```python
from build123d import *

# Parameters (mm, degrees)
CROQUIS1_W              = 200
CROQUIS1_H              = 200
CROQUIS1_R              = 2.5
SALIENTE_EXTRUIR1_DEPTH = 0.5
CORTAR_EXTRUIR1_DEPTH   = 10


with BuildPart() as part:
    # Croquis1 → Saliente-Extruir1 (new body)
    with BuildSketch(Plane(origin=(0, 0, 0), x_dir=(1, 0, 0), z_dir=(0, 1, 0))):
        with Locations((100, 100)):
            Rectangle(CROQUIS1_W, CROQUIS1_H)
        with Locations(Location((15, 185, 0), (0, 0, 270))):
            Circle(CROQUIS1_R, mode=Mode.SUBTRACT)
        with Locations(Location((185, 185, 0), (0, 0, 270))):
            Circle(CROQUIS1_R, mode=Mode.SUBTRACT)
        with Locations(Location((185, 15, 0), (0, 0, 270))):
            Circle(CROQUIS1_R, mode=Mode.SUBTRACT)
        with Locations(Location((15, 15, 0), (0, 0, 270))):
            Circle(CROQUIS1_R, mode=Mode.SUBTRACT)
    extrude(amount=SALIENTE_EXTRUIR1_DEPTH)

    # Croquis2 → Cortar-Extruir1 (cut)
    with BuildSketch(Plane(origin=(0, 0.5, 0), x_dir=(1, 0, 0), z_dir=(0, 1, 0))):
        Polygon((50, 148), (50, 100), (50, 52), (52, 52), (52, 50), (100, 50), (148, 50), (148, 52), (150, 52), (150, 100), (150, 148), (148, 148), (148, 150), (100, 150), (52, 150), (52, 148), align=None)
    extrude(amount=-CORTAR_EXTRUIR1_DEPTH, mode=Mode.SUBTRACT)


solid = part.part
```
Geometry check sheet. Reference: the model listing, model coordinates, mm. Give positions to 0.01 mm unless a question says otherwise; leave off trailing zeros. Write each loop counter-clockwise with the first axis right and the second up, starting at its lowest first coordinate (ties: lowest second). Pieces come first, ordered by that corner, then holes. Notation, with made-up numbers: (-37, 7) -> (-30, 7) arc R24 ccw to (-30, 41) -> close; hole circle Ø10 at (-34, -9.5). An arc over 180 degrees is marked (long way). One line per question, with ' | ' between items.
Item 1: Sectioned sample at A-A, the plane z = -106. Record the boundary of the cut face in (x, y).
Determined:
outline: (0, 0) -> (50, 0) -> (50, 0.5) -> (0, 0.5) -> close; (150, 0) -> (200, 0) -> (200, 0.5) -> (150, 0.5) -> close
Item 2: Sectioned sample at C-C, the plane y = 0.3. Record the boundary of the cut face in (x, z), plus the area to 3 significant figures.
Determined:
outline: (0, -200) -> (200, -200) -> (200, 0) -> (0, 0) -> close; hole circle Ø5 at (15, -185); hole circle Ø5 at (15, -15); hole (50, -148) -> (52, -148) -> (52, -150) -> (148, -150) -> (148, -148) -> (150, -148) -> (150, -52) -> (148, -52) -> (148, -50) -> (52, -50) -> (52, -52) -> (50, -52) -> close; hole circle Ø5 at (185, -185); hole circle Ø5 at (185, -15) | area: 29,900 mm^2
Item 3: Draft check along X on faces 1 (the flat face through (99, 0.5, -35)), 2 (the cylindrical face through (13.5, 0.2, -17)). Enter one of: released by +X, released by -X, zero draft, split by the parting line, or undercut.
Determined:
face 1: zero draft | face 2: undercut
Item 4: Scan lines: line 1 along Z through (x, y) = (185, 0.25); line 2 along X through (y, z) = (0.45, -15); line 3 along X through (y, z) = (0.1, -94.5). Record each from-to range of solid material in increasing order.
Determined:
line 1: -200 to -187.5, -182.5 to -17.5, -12.5 to 0 | line 2: 0 to 12.5, 17.5 to 182.5, 187.5 to 200 | line 3: 0 to 50, 150 to 200
Item 5: Depth check by flat-ended pin: pin 1 (3 mm diameter, centred on x = 185, z = -185, fed in from -Y); pin 2 (6.5 mm diameter, centred on x = 15, z = -185, fed in from -Y). Enter the tip coordinate at first touch or a pass-through.
Determined:
pin 1: through | pin 2: y = 0
Item 6: Sectioned sample at D-D, the plane z = -15. Record the boundary of the cut face in (x, y).
Determined:
outline: (0, 0) -> (12.5, 0) -> (12.5, 0.5) -> (0, 0.5) -> close; (17.5, 0) -> (182.5, 0) -> (182.5, 0.5) -> (17.5, 0.5) -> close; (187.5, 0) -> (200, 0) -> (200, 0.5) -> (187.5, 0.5) -> close
Item 7: Sectioned sample at B-B, the plane x = 15. Record the boundary of the cut face in (y, z), plus the area to 3 significant figures.
Determined:
outline: (0, -200) -> (0.5, -200) -> (0.5, -187.5) -> (0, -187.5) -> close; (0, -182.5) -> (0.5, -182.5) -> (0.5, -17.5) -> (0, -17.5) -> close; (0, -12.5) -> (0.5, -12.5) -> (0.5, 0) -> (0, 0) -> close | area: 95.0 mm^2
